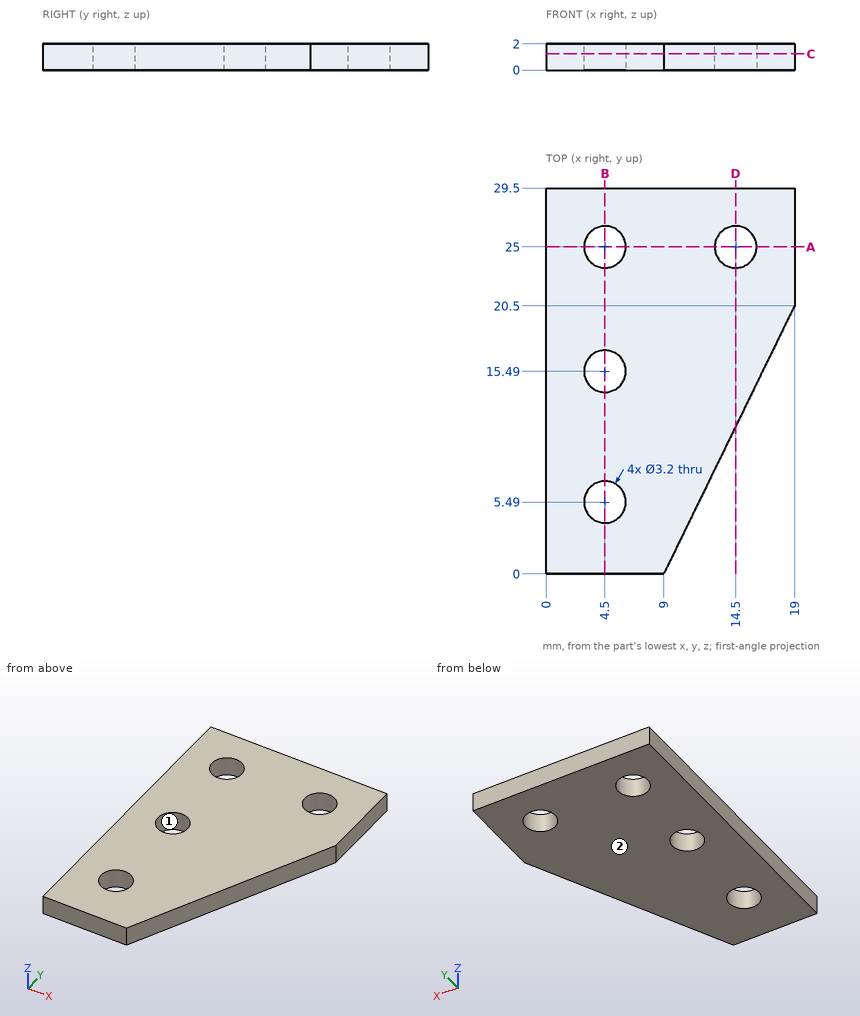
Here's the drawing with two shaded views (mm, measured from the low corner). I have some questions. Give positions to 0.01 mm unless a question says otherwise; leave off trailing zeros. Loops run counter-clockwise (first coordinate to the right, second up) from the corner with the lowest first, then second, coordinate; pieces in that order, holes last. Notation, with made-up numbers: (83, 70) -> (107, 70) arc R29 ccw to (107, 104) -> close; hole circle Ø8 at (-18, 41.5). An arc over 180 degrees is marked (long way). Answer as a JSON object with one key per item and string values. Group by question number.
Item 1: Imagine slicing it at D-D on x = 14.5. Write out the boundary of the cut face in (y, z) (3 decimals), then the cut area to 4 significant figures.
Item 2: Will this pin go through, and if not, where does the flat tip stop? pin 1 (3 mm diameter, centred on x = 14.5, y = 25, fed in from +Z).
Item 3: Imagine slicing it at C-C on z = 1.25. Write out the boundary of the cut face in (x, y), then the cut area to 3 significant figures.
Item 4: I need wall thicknesses on L1, parallel to Y at x = 4.5, z = 0.55; L2, parallel to Y at x = 3.25, z = 1.3; L3, parallel to Y at x = 14.5, z = 1.4 (3 decimals). Which ranges of each line are inside material? Lowest first, please.
Item 5: Thinking about a two-plate mould opening in X: for the marked faces 1 and 2, which applies, pulls with the +X half, pulls with the -X half, needs draft (parallel to the pull), parting line crosses it, or undercut?
Item 6: Imagine slicing it at B-B on x = 4.5. Write out the boundary of the cut face in (y, z), then the cut area to 3 significant figures.
Item 7: Imagine slicing it at A-A on y = 25. Write out the boundary of the cut face in (x, z), then the cut area to 3 significant figures.
Answer list:
{
 "1": {"outline": "(11.275, 0) -> (23.4, 0) -> (23.4, 2) -> (11.275, 2) -> close; (26.6, 0) -> (29.5, 0) -> (29.5, 2) -> (26.6, 2) -> close", "area": "30.05 mm2"},
 "2": {"pin 1": "passes through"},
 "3": {"outline": "(0, 0) -> (9, 0) -> (19, 20.5) -> (19, 29.5) -> (0, 29.5) -> close; hole circle Ø3.2 at (4.5, 5.49); hole circle Ø3.2 at (4.5, 15.49); hole circle Ø3.2 at (4.5, 25); hole circle Ø3.2 at (14.5, 25)", "area": "426 mm2"},
 "4": {"L1": "y = 0 to 3.89, 7.09 to 13.89, 17.09 to 23.4, 26.6 to 29.5", "L2": "y = 0 to 4.49, 6.49 to 14.49, 16.49 to 24, 26 to 29.5", "L3": "y = 11.275 to 23.4, 26.6 to 29.5"},
 "5": {"face 1": "undercut", "face 2": "needs draft"},
 "6": {"outline": "(0, 0) -> (3.89, 0) -> (3.89, 2) -> (0, 2) -> close; (7.09, 0) -> (13.89, 0) -> (13.89, 2) -> (7.09, 2) -> close; (17.09, 0) -> (23.4, 0) -> (23.4, 2) -> (17.09, 2) -> close; (26.6, 0) -> (29.5, 0) -> (29.5, 2) -> (26.6, 2) -> close", "area": "39.8 mm2"},
 "7": {"outline": "(0, 0) -> (2.9, 0) -> (2.9, 2) -> (0, 2) -> close; (6.1, 0) -> (12.9, 0) -> (12.9, 2) -> (6.1, 2) -> close; (16.1, 0) -> (19, 0) -> (19, 2) -> (16.1, 2) -> close", "area": "25.2 mm2"}
}
